Source: CAD feature listing. Evaluate the final solid. Frame: model axes, mm. Give positions to 0.01 mm unless a question says otherwise; leave off trailing zeros. Write each loop counter-clockwise with the first axis right and the second up, starting at its lowest first coordinate (ties: lowest second). Pieces come first, ordered by that corner, then holes. Notation, with made-up numbers: (49.25, 6) -> (59.25, 6) arc R14 cw to (59.25, 11) -> close; hole circle Ø4 at (66.5, 25.25). An arc over 180 degrees is marked (long way). Write item = value, one per line.
from build123d import *

# Parameters (mm, degrees)
F0_R     = 10
F1_DEPTH = 150
F3_DEPTH = 15


with BuildPart() as f1:
    # F0 (on Front) → F1 (new body, symmetric)
    with BuildSketch(Plane.XZ):
        Circle(F0_R)
    extrude(amount=F1_DEPTH, both=True)

    # F2 (on face) → F3 (cut)
    with BuildSketch(Plane.XZ.offset(150)):
        with BuildLine():
            Line((-1, 8.4674081294), (-1, 9.9498743711))
            ThreePointArc((-1, 9.9498743711), (-2.588190451, 9.6592582629), (-4.1089117817, 9.1168439698))
            Line((-4.1089117817, 9.1168439698), (-3.3676786609, 7.8329905443))
            ThreePointArc((-3.3676786609, 7.8329905443), (-2.2067568147, 8.2357285525), (-1, 8.4674081294))
        make_face()
        with BuildLine():
            Line((3.3676786609, 7.8329905443), (4.1089117817, 9.1168439698))
            ThreePointArc((4.1089117817, 9.1168439698), (2.588190451, 9.6592582629), (1, 9.9498743711))
            Line((1, 9.9498743711), (1, 8.4674081294))
            ThreePointArc((1, 8.4674081294), (2.2067568147, 8.2357285525), (3.3676786609, 7.8329905443))
        make_face()
        with BuildLine():
            Line((6.8329905443, 5.0997294685), (8.1168439698, 5.8409625893))
            ThreePointArc((8.1168439698, 5.8409625893), (7.0710678119, 7.0710678119), (5.8409625893, 8.1168439698))
            Line((5.8409625893, 8.1168439698), (5.0997294685, 6.8329905443))
            ThreePointArc((5.0997294685, 6.8329905443), (6.0289717378, 6.0289717378), (6.8329905443, 5.0997294685))
        make_face()
        with BuildLine():
            Line((8.4674081294, 1), (9.9498743711, 1))
            ThreePointArc((9.9498743711, 1), (9.6592582629, 2.588190451), (9.1168439698, 4.1089117817))
            Line((9.1168439698, 4.1089117817), (7.8329905443, 3.3676786609))
            ThreePointArc((7.8329905443, 3.3676786609), (8.2357285525, 2.2067568147), (8.4674081294, 1))
        make_face()
        with BuildLine():
            ThreePointArc((9.1168439698, -4.1089117817), (9.6592582629, -2.588190451), (9.9498743711, -1))
            Line((9.9498743711, -1), (8.4674081294, -1))
            ThreePointArc((8.4674081294, -1), (8.2357285525, -2.2067568147), (7.8329905443, -3.3676786609))
            Line((7.8329905443, -3.3676786609), (9.1168439698, -4.1089117817))
        make_face()
        with BuildLine():
            ThreePointArc((5.8409625893, -8.1168439698), (7.0710678119, -7.0710678119), (8.1168439698, -5.8409625893))
            Line((8.1168439698, -5.8409625893), (6.8329905443, -5.0997294685))
            ThreePointArc((6.8329905443, -5.0997294685), (6.0289717378, -6.0289717378), (5.0997294685, -6.8329905443))
            Line((5.0997294685, -6.8329905443), (5.8409625893, -8.1168439698))
        make_face()
        with BuildLine():
            ThreePointArc((1, -9.9498743711), (2.588190451, -9.6592582629), (4.1089117817, -9.1168439698))
            Line((4.1089117817, -9.1168439698), (3.3676786609, -7.8329905443))
            ThreePointArc((3.3676786609, -7.8329905443), (2.2067568147, -8.2357285525), (1, -8.4674081294))
            Line((1, -8.4674081294), (1, -9.9498743711))
        make_face()
        with BuildLine():
            ThreePointArc((-4.1089117817, -9.1168439698), (-2.588190451, -9.6592582629), (-1, -9.9498743711))
            Line((-1, -9.9498743711), (-1, -8.4674081294))
            ThreePointArc((-1, -8.4674081294), (-2.2067568147, -8.2357285525), (-3.3676786609, -7.8329905443))
            Line((-3.3676786609, -7.8329905443), (-4.1089117817, -9.1168439698))
        make_face()
        with BuildLine():
            ThreePointArc((-8.1168439698, -5.8409625893), (-7.0710678119, -7.0710678119), (-5.8409625893, -8.1168439698))
            Line((-5.8409625893, -8.1168439698), (-5.0997294685, -6.8329905443))
            ThreePointArc((-5.0997294685, -6.8329905443), (-6.0289717378, -6.0289717378), (-6.8329905443, -5.0997294685))
            Line((-6.8329905443, -5.0997294685), (-8.1168439698, -5.8409625893))
        make_face()
        with BuildLine():
            ThreePointArc((-9.9498743711, -1), (-9.6592582629, -2.588190451), (-9.1168439698, -4.1089117817))
            Line((-9.1168439698, -4.1089117817), (-7.8329905443, -3.3676786609))
            ThreePointArc((-7.8329905443, -3.3676786609), (-8.2357285525, -2.2067568147), (-8.4674081294, -1))
            Line((-8.4674081294, -1), (-9.9498743711, -1))
        make_face()
        with BuildLine():
            Line((-7.8329905443, 3.3676786609), (-9.1168439698, 4.1089117817))
            ThreePointArc((-9.1168439698, 4.1089117817), (-9.6592582629, 2.588190451), (-9.9498743711, 1))
            Line((-9.9498743711, 1), (-8.4674081294, 1))
            ThreePointArc((-8.4674081294, 1), (-8.2357285525, 2.2067568147), (-7.8329905443, 3.3676786609))
        make_face()
        with BuildLine():
            Line((-5.0997294685, 6.8329905443), (-5.8409625893, 8.1168439698))
            ThreePointArc((-5.8409625893, 8.1168439698), (-7.0710678119, 7.0710678119), (-8.1168439698, 5.8409625893))
            Line((-8.1168439698, 5.8409625893), (-6.8329905443, 5.0997294685))
            ThreePointArc((-6.8329905443, 5.0997294685), (-6.0289717378, 6.0289717378), (-5.0997294685, 6.8329905443))
        make_face()
    extrude(amount=-F3_DEPTH, mode=Mode.SUBTRACT)


solid = f1.part
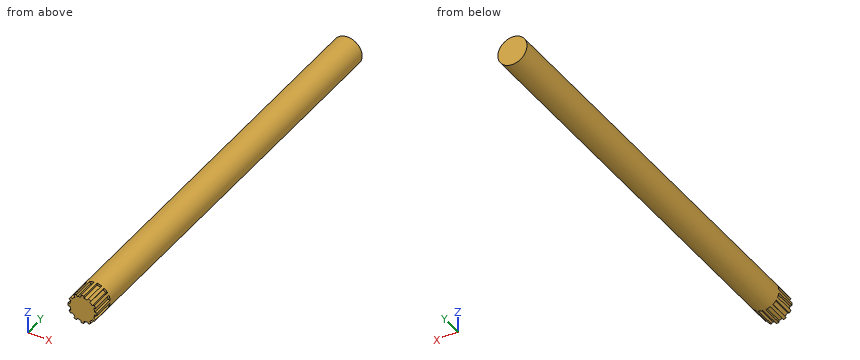
(1) Section query A-A (y = -88). Return loops of the section in (x, z).
Values follow:
outline = circle Ø20 at (0, 0)
(2) Material intervals for line 1 (Y direction, x = 7.75, z = -5.75); line 2 (X direction, y = 123, z = 0.25); line 3 (X direction, y = 115, z = -4), sorted ascending.
Values follow:
line_1 = -135 to 150
line_2 = -10 to 10
line_3 = -9.17 to 9.17
(3) First-contact query: pin 1 (1.2 mm diameter, centred on x = -9.5, y = -139.5, fed in from +Z); pin 2 (3 mm diameter, centred on y = -2, z = -8, fed in from +X); pin 3 (0.7 mm diameter, centred on y = -141.5, z = -9.5, fed in from +X). Flat tips, straight axial feed; report the tip coordinate or a pass-through.
Values follow:
pin_1 = 4.56
pin_2 = 7.6
pin_3 = 1
